from build123d import *

# Parameters (mm, degrees)
F1_DEPTH        = 15
F2_DEPTH        = 20
F3_DEPTH        = 5
F5_DEPTH        = 5
F5_COPIES_COUNT = 4


# Not quite as in the source:
# - a pattern or mirror of a feature is missing from the dataset's text; its kind, count and spacing are read off the source's solid


with BuildPart() as f1:
    # F0 (on Front) → F1 (new body)
    with BuildSketch(Plane.XZ):
        Polygon((-4.1421356237, -1.7157287525), (-1.7157287525, -4.1421356237), (1.7157287525, -4.1421356237), (4.1421356237, -1.7157287525), (4.1421356237, 1.7157287525), (1.7157287525, 4.1421356237), (-1.7157287525, 4.1421356237), (-4.1421356237, 1.7157287525), align=None)
    extrude(amount=F1_DEPTH)

    # F0 (on Front) → F2 (join)
    with BuildSketch(Plane.XZ):
        Polygon((4.1421356237, -10), (10, -4.1421356237), (10, 4.1421356237), (4.1421356237, 10), (-4.1421356237, 10), (-10, 4.1421356237), (-10, -4.1421356237), (-4.1421356237, -10), align=None)
        Polygon((1.7157287525, -4.1421356237), (-1.7157287525, -4.1421356237), (-4.1421356237, -1.7157287525), (-4.1421356237, 1.7157287525), (-1.7157287525, 4.1421356237), (1.7157287525, 4.1421356237), (4.1421356237, 1.7157287525), (4.1421356237, -1.7157287525), align=None, mode=Mode.SUBTRACT)
    extrude(amount=F2_DEPTH)

    # F0 (on Front) → F3 (cut)
    with BuildSketch(Plane.XZ):
        Polygon((-4.1421356237, -1.7157287525), (-1.7157287525, -4.1421356237), (1.7157287525, -4.1421356237), (4.1421356237, -1.7157287525), (4.1421356237, 1.7157287525), (1.7157287525, 4.1421356237), (-1.7157287525, 4.1421356237), (-4.1421356237, 1.7157287525), align=None)
    extrude(amount=F3_DEPTH, mode=Mode.SUBTRACT)

    # F4 (on face) → F5 (cut)
    with BuildSketch(Plane(origin=(0, 0, -10), x_dir=(1, 0, 0), z_dir=(0, 0, -1))):
        Polygon((-4.1421356237, 11.7157287525), (-4.1421356237, 8.2842712475), (-1.7157287525, 5.8578643763), (1.7157287525, 5.8578643763), (4.1421356237, 8.2842712475), (4.1421356237, 11.7157287525), (1.7157287525, 14.1421356237), (-1.7157287525, 14.1421356237), align=None)
    f5 = extrude(amount=-F5_DEPTH, mode=Mode.SUBTRACT)

    # F5_copies: F5 ×4 about axis
    f5_copies_axis = Axis((0, 0, 0), (0, 1, 0))
    for i in range(1, F5_COPIES_COUNT):
        add(f5.rotate(f5_copies_axis, i * 360 / F5_COPIES_COUNT), mode=Mode.SUBTRACT)


solid = f1.part
Could you check a few things on this model? Use its own coordinates, in mm. A direction names the side the tool comes from. Give positions to 0.01 mm unless a question says otherwise; leave off trailing zeros. Order: outer loops, then holes, each group sorted by start corner. A loop starts at its lowest first (then second) coordinate and runs counter-clockwise, first axis right, second up.
Item 1: For faces 1 (the face through (-2.95, -17.46, 2.91)), 2 (the face through (0, -5.858, 8)), 3 (the face through (7.53, -12.91, 2.95)), 4 (the face through (-2.91, -12.95, -7.54)), 5 (the face through (4.142, -2, 0)), which set-ups out of +Z, -Z, +X, -X, +Y, -Y let a thin tool reach every point of the face, with its end or its side?
Item 2: If we section it at A-A, the plane y = -18.25: Write out the boundary of the cut face in (x, z).
Item 3: If we section it at C-C, the plane z = -0.25: Write out the boundary of the cut face in (x, y).
Item 4: If we section it at D-D, the plane x = -6: Write out the boundary of the cut face in (y, z).
Item 5: I need wall thicknesses on line 1 (Y direction, x = 1, z = 6); line 2 (X direction, y = -13.5, z = 0.5); line 3 (Z direction, x = -0.5, y = -1.25). Which ranges of each line are inside material? Lowest first, please.
Item 6: I'm going to push flat-ended pins straight in: pin 1 (4 mm diameter, centred on x = 1, z = -0.5, fed in from +Y); pin 2 (2.5 mm diameter, centred on x = 6.5, y = -9.5, fed in from -Z); pin 3 (2 mm diameter, centred on x = -2, z = 3, fed in from +Y); pin 4 (1 mm diameter, centred on x = 7.5, y = -10.5, fed in from +Z). Where does each tip first touch, or does it pass through?
Item 7: If we section it at B-B, the plane x = -0.25: Write out the boundary of the cut face in (y, z), plus the area to 3 significant figures.
Item 8: If we mould it in two halves opening along Z, with no side actions, what happens to faces 6 (the face through (0, -17, -10)), 7 (the face through (7.53, -7.05, 2.91)), 8 (the face through (0, -14.142, -8))? For each: pulls with the +Z half, pulls with the -Z half, needs draft (parallel to the pull), parting line crosses it, or undercut.
Values:
1. face 1: -Y
1. face 2: +Z
1. face 3: +X
1. face 4: -Z
1. face 5: +Y
2. outline: (-10, -4.14) - (-4.14, -10) - (4.14, -10) - (10, -4.14) - (10, 4.14) - (4.14, 10) - (-4.14, 10) - (-10, 4.14) - close; hole (-4.14, -1.72) - (-1.72, -4.14) - (1.72, -4.14) - (4.14, -1.72) - (4.14, 1.72) - (1.72, 4.14) - (-1.72, 4.14) - (-4.14, 1.72) - close
3. outline: (-10, -20) - (-4.14, -20) - (-4.14, -15) - (4.14, -15) - (4.14, -20) - (10, -20) - (10, -14.14) - (5, -14.14) - (5, -5.86) - (10, -5.86) - (10, 0) - (4.14, 0) - (4.14, -5) - (-4.14, -5) - (-4.14, 0) - (-10, 0) - (-10, -5.86) - (-5, -5.86) - (-5, -14.14) - (-10, -14.14) - close
4. outline: (-20, -8.14) - (0, -8.14) - (0, 8.14) - (-20, 8.14) - close; hole (-14.14, -1.72) - (-11.72, -4.14) - (-8.28, -4.14) - (-5.86, -1.72) - (-5.86, 1.72) - (-8.28, 4.14) - (-11.72, 4.14) - (-14.14, 1.72) - close
5. line 1: y = -20 to -14.14, -5.86 to 0
5. line 2: x = -5 to 5
5. line 3: z = -10 to -4.14, 4.14 to 10
6. pin 1: stops at y = -5
6. pin 2: stops at z = -8.89
6. pin 3: stops at y = 0
6. pin 4: stops at z = 7.14
7. outline: (-20, -10) - (-14.14, -10) - (-14.14, -5) - (-5.86, -5) - (-5.86, -10) - (0, -10) - (0, -4.14) - (-5, -4.14) - (-5, 4.14) - (0, 4.14) - (0, 10) - (-5.86, 10) - (-5.86, 5) - (-14.14, 5) - (-14.14, 10) - (-20, 10) - (-20, 4.14) - (-15, 4.14) - (-15, -4.14) - (-20, -4.14) - close
7. area: 234 mm2
8. face 6: pulls with the -Z half
8. face 7: undercut
8. face 8: needs draft
